```python
from build123d import *

# Parameters (mm, degrees)
F0_W     = 88
F0_H     = 88
F1_DEPTH = 9


with BuildPart() as f1:
    # F0 (on Top) → F1 (new body)
    with BuildSketch(Plane.XY):
        Rectangle(F0_W, F0_H)
        with BuildLine():
            ThreePointArc((-34, 17.5), (-32.039498, 22.152199), (-27.340629, 23.998046))
            Line((-27.340629, 23.998046), (8.217317, 24))
            ThreePointArc((8.217317, 24), (12.813742, 22.09632), (14.717675, 17.5))
            Line((14.717675, 17.5), (14.717675, -15.522273))
            ThreePointArc((14.717675, -15.522273), (13.127514, -19.781789), (9.135066, -21.957209))
            ThreePointArc((9.135066, -21.957209), (8.229219, -22.022263), (7.323146, -21.960427))
            Line((7.323146, -21.960427), (-27.476912, -22.022232))
            ThreePointArc((-27.476912, -22.022232), (-27.488456, -22.022263), (-27.5, -22.022273))
            ThreePointArc((-27.5, -22.022273), (-32.096194, -20.118467), (-34, -15.522273))
            Line((-34, -15.522273), (-34, 17.5))
        make_face(mode=Mode.SUBTRACT)
    extrude(amount=F1_DEPTH)


solid = f1.part
```
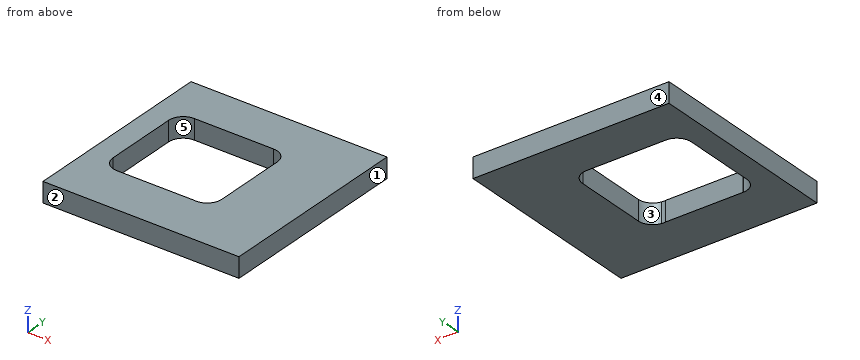
Verification items for the finished model (mm, model axes). Face numbers are marked on the shaded views. A direction names the side the tool comes from. Give positions to 0.01 mm unless a question says otherwise; leave off trailing zeros. Loops run counter-clockwise (first coordinate to the right, second up) from the corner with the lowest first, then second, coordinate; pieces in that order, holes last.
1. Thickness scan on line 1 (Y direction, x = -26.5, z = 0.5); line 2 (X direction, y = -13.5, z = 6.75); line 3 (Y direction, x = -31.5, z = 1). Record the ranges inside material, lowest first.
2. Section check C-C, the plane x = -9. Enter the section's corners in (y, z).
3. Mould release check, pull along Y, two halves, no side actions. Record for the marked faces 1, 2 and 3: released by +Y, released by -Y, zero draft, split by the parting line, or undercut.
4. Go/stop test with a flat-tipped pin: pin 1 Ø12 at (x, y) = (-29.5, -32) entering from -Z. Record where the tip stops, or that it passes through.
5. Set-up check for the marked faces 4 and 5: record each of +Z, -Z, +X, -X, +Y, -Y from which the full face is reachable in a straight line by a thin tool's end or side.
6. Section check B-B, the plane y = 4.5. Enter the section's corners in (x, z).
Geometry says:
1. line 1: y = -44 to -22.02, 24 to 44
1. line 2: x = -44 to -34, 14.72 to 44
1. line 3: y = -44 to -20.65, 22.62 to 44
2. outline: (-44, 0) - (-21.99, 0) - (-21.99, 9) - (-44, 9) - close; (24, 0) - (44, 0) - (44, 9) - (24, 9) - close
3. face 1: zero draft
3. face 2: released by -Y
3. face 3: undercut
4. pin 1: stops at z = 0
5. face 4: +Z, -Z, +X, -X, +Y
5. face 5: +Z, -Z
6. outline: (-44, 0) - (-34, 0) - (-34, 9) - (-44, 9) - close; (14.72, 0) - (44, 0) - (44, 9) - (14.72, 9) - close
